```python
from build123d import *

# Parameters (mm, degrees)
SKETCH1_W                = 50
SKETCH1_H                = 100
BASE_FLANGE1_DEPTH       = 2
SKETCHED_START           = -25
SKETCHED_BEND1_DEPTH     = 50
SKETCHED_BEND1_2_DEPTH   = 50
CUT_EXTRUDE2_DEPTH       = 60.702826072
BOSS_EXTRUDE2_DEPTH      = 75
BOSS_EXTRUDE2_DEPTH_BACK = 75
SKETCH9_R                = 5
SKETCH10_R               = 1.75
CUT_EXTRUDE3_DEPTH       = 116.029027735
SKETCH11_R               = 2.61136214
CUT_EXTRUDE4_DEPTH       = 161.886846393


# Read off the part's stored shape, not the designer's step: Sketched Bend1
# Sheet-metal steps are written as plain solids
with BuildPart() as part:
    # Sketch1 → Base-Flange1 (new body)
    with BuildSketch(Plane(origin=(0, 0, 0), x_dir=(1, 0, 0), z_dir=(0, 1, 0))):
        Rectangle(SKETCH1_W, SKETCH1_H)
    extrude(amount=-BASE_FLANGE1_DEPTH)

    # Sketched Bend1 outline → Sketched Bend1 (cut)
    with BuildSketch(Plane.YZ.offset(SKETCHED_START)):
        with BuildLine():
            Line((0, -50), (0, -30.905812394))
            Line((0, -30.905812394), (-0.02606043, -30.896327173))
            ThreePointArc((-0.02606043, -30.896327173), (-1.457456133, -29.79797862), (-2, -28.077249311))
            Line((-2, -28.077249311), (-2, -50))
            Line((-2, -50), (0, -50))
        make_face()
    extrude(amount=SKETCHED_BEND1_DEPTH, mode=Mode.SUBTRACT)

    # Sketched Bend1 2 outline → Sketched Bend1 2 (add)
    with BuildSketch(Plane.YZ.offset(SKETCHED_START)):
        with BuildLine():
            Line((0, -30.905812394), (18.278484393, -37.558636641))
            Line((18.278484393, -37.558636641), (18.96252468, -35.679251399))
            Line((18.96252468, -35.679251399), (0.657979857, -29.016941932))
            ThreePointArc((0.657979857, -29.016941932), (0.180847956, -28.650825747), (0, -28.077249311))
            Line((0, -28.077249311), (0, -30.905812394))
        make_face()
    extrude(amount=SKETCHED_BEND1_2_DEPTH)

    # Sketch8 → Cut-Extrude2 (cut, through all)
    with BuildSketch(Plane.XZ.offset(2)):
        with BuildLine():
            Line((-25, 45), (-25, -23.077249311))
            ThreePointArc((-25, -23.077249311), (-9.62789438, 10.961375345), (-25, 45))
        make_face()
        with BuildLine():
            Line((25, -23.077249311), (25, 45))
            ThreePointArc((25, 45), (9.62789438, 10.961375345), (25, -23.077249311))
        make_face()
    extrude(amount=-CUT_EXTRUDE2_DEPTH, mode=Mode.SUBTRACT)

    # Sketch9 → Boss-Extrude2 (add, two sides: drawn at the far end of the back side and taken through both)
    with BuildSketch(Plane(origin=(0, 0, 0), x_dir=(0, 0, -1), z_dir=(1, 0, 0)).offset(-BOSS_EXTRUDE2_DEPTH_BACK)):
        with Locations((-50, -1)):
            Circle(SKETCH9_R)
    extrude(amount=BOSS_EXTRUDE2_DEPTH + BOSS_EXTRUDE2_DEPTH_BACK)

    # Sketch10 → Cut-Extrude3 (cut, through all)
    with BuildSketch(Plane(origin=(0, -9.932936637, -27.290519119), x_dir=(-1, 0, 0), z_dir=(0, -0.34202014332566616, -0.9396926207859094))):
        with Locations(Location((-20, 15.542677454, 0), (0, 0, 90))):
            Circle(SKETCH10_R)
        with Locations(Location((-12, 15.542677454, 0), (0, 0, 90))):
            Circle(SKETCH10_R)
        with Locations(Location((-4, 15.542677454, 0), (0, 0, 90))):
            Circle(SKETCH10_R)
        with Locations(Location((4, 15.542677454, 0), (0, 0, 90))):
            Circle(SKETCH10_R)
        with Locations(Location((12, 15.542677454, 0), (0, 0, 90))):
            Circle(SKETCH10_R)
        with Locations(Location((20, 15.542677454, 0), (0, 0, 90))):
            Circle(SKETCH10_R)
    extrude(amount=-CUT_EXTRUDE3_DEPTH, mode=Mode.SUBTRACT)

    # Sketch11 → Cut-Extrude4 (cut, through all)
    with BuildSketch(Plane.ZY.offset(75)):
        with Locations((50, -1)):
            Circle(SKETCH11_R)
    extrude(amount=-CUT_EXTRUDE4_DEPTH, mode=Mode.SUBTRACT)


solid = part.part
```
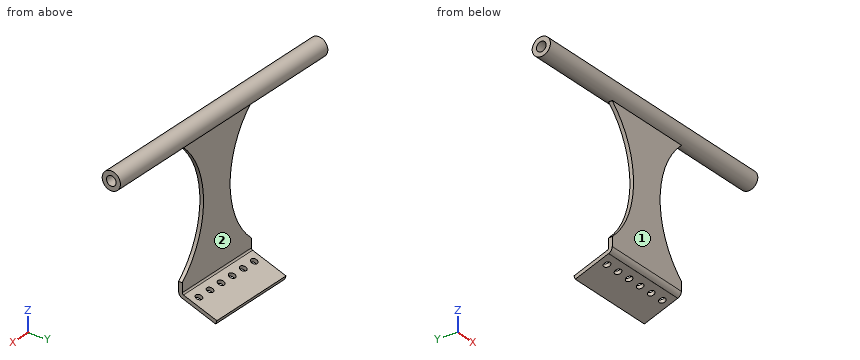
Work out the finished part from the listing and answer in its coordinate system (mm). Face numbers are marked on the shaded views. Give positions to 0.01 mm unless a question says otherwise; leave off trailing zeros. Loops run counter-clockwise (first coordinate to the right, second up) from the corner with the lowest first, then second, coordinate; pieces in that order, holes last. Notation, with made-up numbers: (-37, -12) - (16, -12) arc R22 ccw to (16, 27) - close; hole circle Ø10 at (-35.5, -5.75). An arc over 180 degrees is marked (long way). Use CSV: the item, a comma, the result in double quotes. Start each with the question number.
(1) Find section B-B, the plane z = 10. Determine the outline of the cut face in (x, y).
(2) Find section C-C, the plane z = 21.5. Determine the outline of the cut face in (x, y).
(3) Determine the mould class of the marked faces 1 and 2 for opening direction Z: released by +Z, released by -Z, zero draft, split by the parting line, or undercut.
(4) Find the intervals of material crossed by L1, parallel to Y at x = 31, z = 50; L2, parallel to Y at x = 15, z = 51.5; L3, parallel to Y at x = 8.5, z = -3, in increasing order.
(5) Each of these flat-tipped pins is pushed along its axis until it touches: pin 1 (15 mm diameter, centred on x = 0.5, z = -9.5, fed in from -Y); pin 2 (3 mm diameter, centred on y = -1.5, z = 11.5, fed in from -X); pin 3 (12 mm diameter, centred on x = 3, y = 14, fed in from -Z); pin 4 (7 mm diameter, centred on y = 13.5, z = -27.5, fed in from +X). Where does it stop, or does it pass through?
(6) Find section A-A, the plane z = 50. Determine the outline of the cut face in (x, y).
Results found:
1,outline,"(-9.64, -2) - (9.64, -2) - (9.64, 0) - (-9.64, 0) - close"
2,outline,"(-10.87, -2) - (10.87, -2) - (10.87, 0) - (-10.87, 0) - close"
3,face 1,"zero draft"
3,face 2,"undercut"
4,L1,"-6 to -3.61, 1.61 to 4"
4,L2,"-5.77 to -3.14, 1.14 to 3.77"
4,L3,"-2 to 0"
5,pin 1,"y = -2"
5,pin 2,"x = -9.67"
5,pin 3,"z = -37.56"
5,pin 4,"through"
6,outline,"(-75, -6) - (75, -6) - (75, -3.61) - (-75, -3.61) - close; (-75, 1.61) - (75, 1.61) - (75, 4) - (-75, 4) - close"
